from build123d import *

# Parameters (mm, degrees)
F0_W     = 292.1
F0_H     = 292.1
F0_R     = 2.06375
F1_DEPTH = 3.175
F2_R     = 1.778
F2_W     = 16.0782
F2_H     = 16.0782
F2_R_2   = 2.06375
F2_R_3   = 12.7
F2_R_4   = 6.0325
F2_R_5   = 2.032
F2_R_6   = 1.651
F2_W_2   = 73.787
F2_H_2   = 4.064
F3_DEPTH = 3.176
F4_R     = 5.08
F5_R     = 1.27
F6_R     = 6.35
F7_R     = 1.778


with BuildPart() as f1:
    # F0 (on Top) → F1 (new body)
    with BuildSketch(Plane.XY):
        Rectangle(F0_W, F0_H)
        with Locations((-133.35, -133.35)):
            Circle(F0_R, mode=Mode.SUBTRACT)
        with Locations((133.35, -133.35)):
            Circle(F0_R, mode=Mode.SUBTRACT)
        with Locations((-133.35, 133.35)):
            Circle(F0_R, mode=Mode.SUBTRACT)
        with Locations((133.35, 133.35)):
            Circle(F0_R, mode=Mode.SUBTRACT)
    extrude(amount=-F1_DEPTH)

    # F2 (on face) → F3 (cut, through all)
    with BuildSketch(Plane.XY):
        with BuildLine():
            Line((-114.6175, -37.7825), (-16.1925, -37.7825))
            Line((-16.1925, -37.7825), (-16.1925, 117.7925))
            Line((-16.1925, 117.7925), (-59.055, 117.7925))
            Line((-59.055, 117.7925), (-59.055, 130.4925))
            ThreePointArc((-59.055, 130.4925), (-65.405, 136.8425), (-71.755, 130.4925))
            Line((-71.755, 130.4925), (-71.755, 117.7925))
            Line((-71.755, 117.7925), (-114.6175, 117.7925))
            Line((-114.6175, 117.7925), (-114.6175, -37.7825))
        make_face()
        with Locations((-116.3955, -91.1225)):
            Circle(F2_R)
        with Locations((-71.9455, -91.1225)):
            Circle(F2_R)
        with Locations((-71.9455, -135.5725)):
            Circle(F2_R)
        with Locations((-116.3955, -135.5725)):
            Circle(F2_R)
        with Locations((-106.5784, -100.9396)):
            Rectangle(F2_W, F2_H)
        with Locations((-81.7626, -100.9396)):
            Rectangle(F2_W, F2_H)
        with Locations((-106.5784, -125.7554)):
            Rectangle(F2_W, F2_H)
        with Locations((-81.7626, -125.7554)):
            Rectangle(F2_W, F2_H)
        with Locations((-129.06375, -32.5755)):
            Circle(F2_R_2)
        with Locations((-1.74625, -32.5755)):
            Circle(F2_R_2)
        with Locations((31.242, -102.108)):
            Circle(F2_R_3)
        with Locations((114.808, -102.108)):
            Circle(F2_R_3)
        with Locations((31.242, 96.012)):
            Circle(F2_R_4)
        with Locations((31.242, 45.212)):
            Circle(F2_R_4)
        with Locations((31.242, -5.588)):
            Circle(F2_R_4)
        with Locations((73.025, 96.012)):
            Circle(F2_R_4)
        with Locations((73.025, 45.212)):
            Circle(F2_R_4)
        with Locations((73.025, -5.588)):
            Circle(F2_R_4)
        with Locations((114.808, 96.012)):
            Circle(F2_R_4)
        with Locations((114.808, 45.212)):
            Circle(F2_R_4)
        with Locations((114.808, -5.588)):
            Circle(F2_R_4)
        with Locations((-43.815, -113.3475)):
            Circle(F2_R_3)
        with Locations((12.51585, -102.108)):
            Circle(F2_R_5)
        with Locations((49.96815, -102.108)):
            Circle(F2_R_5)
        with Locations((96.08185, -102.108)):
            Circle(F2_R_5)
        with Locations((133.53415, -102.108)):
            Circle(F2_R_5)
        with Locations((-129.06375, 112.5855)):
            Circle(F2_R_2)
        with Locations((-1.74625, 112.5855)):
            Circle(F2_R_2)
        with Locations((-129.06375, 40.005)):
            Circle(F2_R_2)
        with Locations((-1.74625, 40.005)):
            Circle(F2_R_2)
        with Locations((33.20415, -52.4891)):
            Circle(F2_R_6)
        with Locations((112.84585, -52.4891)):
            Circle(F2_R_6)
        with Locations((-88.265, -61.75375)):
            Circle(F2_R_2)
        with Locations((-43.815, -61.75375)):
            Circle(F2_R_2)
        with Locations((73.025, -52.4891)):
            Rectangle(F2_W_2, F2_H_2)
    extrude(amount=-F3_DEPTH, mode=Mode.SUBTRACT)

    # F4
    f4_edges = [f1.edges().sort_by_distance(p)[0] for p in [
        (-114.6175, 117.7925, -1.5875),
        (-16.1925, 117.7925, -1.5875),
        (-16.1925, -37.7825, -1.5875),
        (-114.6175, -37.7825, -1.5875),
        (-59.055, 117.7925, -1.5875),
        (-71.755, 117.7925, -1.5875),
    ]]
    fillet(f4_edges, radius=F4_R)

    # F5
    f5_edges = [f1.edges().sort_by_distance(p)[0] for p in [
        (-114.6175, -92.9005, -1.5875),
        (-89.8017, -92.9005, -1.5875),
        (-89.8017, -117.7163, -1.5875),
        (-114.6175, -117.7163, -1.5875),
        (-98.5393, -92.9005, -1.5875),
        (-73.7235, -92.9005, -1.5875),
        (-98.5393, -117.7163, -1.5875),
        (-73.7235, -117.7163, -1.5875),
        (-73.7235, -133.7945, -1.5875),
        (-73.7235, -108.9787, -1.5875),
        (-98.5393, -108.9787, -1.5875),
        (-98.5393, -133.7945, -1.5875),
        (-114.6175, -133.7945, -1.5875),
        (-114.6175, -108.9787, -1.5875),
        (-89.8017, -108.9787, -1.5875),
        (-89.8017, -133.7945, -1.5875),
    ]]
    fillet(f5_edges, radius=F5_R)

    # F6
    f6_edges = [f1.edges().sort_by_distance(p)[0] for p in [
        (-146.05, 146.05, -1.5875),
        (146.05, 146.05, -1.5875),
        (146.05, -146.05, -1.5875),
        (-146.05, -146.05, -1.5875),
    ]]
    fillet(f6_edges, radius=F6_R)

    # F7
    f7_edges = [f1.edges().sort_by_distance(p)[0] for p in [
        (36.1315, -50.4571, -1.5875),
        (109.9185, -50.4571, -1.5875),
        (109.9185, -54.5211, -1.5875),
        (36.1315, -54.5211, -1.5875),
    ]]
    fillet(f7_edges, radius=F7_R)


solid = f1.part
Geometry check sheet. Reference: the model listing, model coordinates, mm. A direction names the side the tool comes from. Round coordinates to 2 decimals unless told otherwise and drop trailing zeros.
Item 1: Access from +Z, -Z, +X, -X, +Y, -Y to the whole of each face (thin tool, end or side, straight path). Record for faces 1 (the face through (144.14, 144.24, -1.61)), 2 (the face through (-65.27, 136.84, -1.57)).
Determined:
face 1: +Z, -Z, +X, +Y
face 2: +Z, -Z
Item 2: Mould release check, pull along Y, two halves, no side actions. Record for faces 3 (the face through (144.14, -144.24, -1.61)), 4 (the face through (-144.24, 144.14, -1.61)), 5 (the face through (34.026, 90.66, -1.565)): +Y half, -Y half, draft (parallel to the pull), parting line (faces both ways), or undercut.
Determined:
face 3: -Y half
face 4: +Y half
face 5: undercut
Item 3: Go/stop test with a flat-tipped pin: pin 1 Ø5.5 at (x, y) = (-71.95, -135.57) entering from -Z (3 decimals). Record where the tip stops, or that it passes through.
Determined:
pin 1: stops at z = -3.175
Item 4: Section check B-B (z = -0.8). Give the number of separate pieces and of enclosed holes in the cut face, plus the area to 3 significant figures.
Determined:
separate pieces: 1
enclosed holes: 40
area: 65,600 mm2
Item 5: Material ranges on line 1 along X through (y, z) = (46, -0.65); line 2 along Y through (x, z) = (-25, -2.9); line 3 along Y through (x, z) = (-2, -3), recorded low to high.
Determined:
line 1: x = -146.05 to -114.62, -16.19 to 25.26, 37.22 to 67.04, 79.01 to 108.83, 120.79 to 146.05
line 2: y = -146.05 to -37.78, 117.79 to 146.05
line 3: y = -146.05 to -34.62, -30.53 to 37.96, 42.05 to 110.54, 114.63 to 146.05
